For this review, take the finished solid that the model builds, in its own axes (mm). Coordinates: 2 decimals unless noted, no trailing zeros. Write each loop counter-clockwise with the first axis right and the second up, starting at its lowest first coordinate (ties: lowest second). Pieces come first, ordered by that corner, then holes. Notation, with made-up numbers: (29.25, -32.75) - (46.25, -32.75) arc R9 ccw to (46.25, -17.75) - close; hole circle Ø1 at (-9.75, 46.25). An arc over 180 degrees is marked (long way). Use one line per item in the form item = value. Start each with the question number.
1) Mouldability with a two-part tool opening along Y and no side actions: class faces 1 (the cylindrical face through (-108.8, 4.8, 0.7)), 2 (the cylindrical face through (108.742, 4.356, 0.685)), 3 (the flat face through (-2, 8, 3)) as pulls with the +Y half, pulls with the -Y half, needs draft (parallel to the pull), parting line crosses it, or undercut.
2) For L1, parallel to Y at x = 0, z = 0.3; L2, parallel to X at y = 2.75, z = 2.2; L3, parallel to X at y = 5, z = 1.2, list the stretches that pass through material, from the lowest coordinate up. Write a range as from..to.
3) We need section A-A (z = 2.2). Give the boundary of the cut face in (x, y).
```python
from build123d import *

# Parameters (mm, degrees)
CROQUIS1_W                                   = 230
CROQUIS1_H                                   = 10
CROQUIS1_R                                   = 1.75
CROQUIS1_R_2                                 = 1.768842751
SALIENTE_EXTRUIR1_DEPTH                      = 3
REFRENTADO_PARA_TORNILLO_TAP_N_CON_C_2_COUNT = 2
REFRENTADO_PARA_TORNILLO_TAP_N_CON_C_2_PITCH = 110.490700251
REFRENTADO_PARA_TORNILLO_TAP_N_CON_C_3_COUNT = 2
REFRENTADO_PARA_TORNILLO_TAP_N_CON_C_3_PITCH = 220.981400502


with BuildPart() as part:
    # Croquis1 → Saliente-Extruir1 (new body)
    with BuildSketch(Plane.XY):
        with Locations((0, 5)):
            Rectangle(CROQUIS1_W, CROQUIS1_H)
        with Locations((0, 4.279276807)):
            Circle(CROQUIS1_R, mode=Mode.SUBTRACT)
        with Locations((-110.490700251, 4.279276807)):
            Circle(CROQUIS1_R_2, mode=Mode.SUBTRACT)
        with Locations((110.490700251, 4.279276807)):
            Circle(CROQUIS1_R, mode=Mode.SUBTRACT)
    extrude(amount=SALIENTE_EXTRUIR1_DEPTH)

    # Croquis3 → Refrentado para tornillo tapón con cabeza plana de clavija de M31 (revolve, cut)
    with BuildSketch(Plane(origin=(-110.490700251, 4.279276807, 3), x_dir=(0, -1, 0), z_dir=(1, 0, 0))):
        Polygon((0, 0), (0, 3), (1.7, 3), (1.7, 1.66), (3.36, 0), align=None)
    refrentado_para_tornillo_tap_n_con_cabez = revolve(axis=Axis((-110.490700251, 4.279276807, 9.35), (0, 0, -1)), mode=Mode.SUBTRACT)

    # Refrentado para tornillo tap_n con c 2: Refrentado para tornillo tapón con cabeza plana de clavija de M31 ×2
    with Locations(*[(i * REFRENTADO_PARA_TORNILLO_TAP_N_CON_C_2_PITCH, 0, 0) for i in range(1, REFRENTADO_PARA_TORNILLO_TAP_N_CON_C_2_COUNT)]):
        add(refrentado_para_tornillo_tap_n_con_cabez, mode=Mode.SUBTRACT)

    # Refrentado para tornillo tap_n con c 3: Refrentado para tornillo tapón con cabeza plana de clavija de M31 ×2
    with Locations(*[(i * REFRENTADO_PARA_TORNILLO_TAP_N_CON_C_3_PITCH, 0, 0) for i in range(1, REFRENTADO_PARA_TORNILLO_TAP_N_CON_C_3_COUNT)]):
        add(refrentado_para_tornillo_tap_n_con_cabez, mode=Mode.SUBTRACT)


solid = part.part
```
Determined:
q1.face_1 = undercut
q1.face_2 = undercut
q1.face_3 = needs draft
q2.L1 = 0..2.53, 6.03..10
q2.L2 = -115..-112.54, -108.44..-2.05, 2.05..108.44, 112.54..115
q2.L3 = -115..-112.11, -108.88..-1.59, 1.59..108.9, 112.09..115
q3.outline = (-115, 0) - (115, 0) - (115, 10) - (-115, 10) - close; hole circle Ø5.12 at (-110.49, 4.28); hole circle Ø5.12 at (0, 4.28); hole circle Ø5.12 at (110.49, 4.28)
